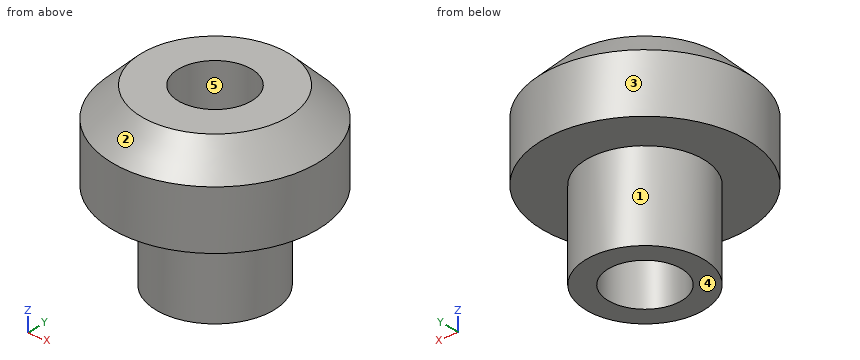
Solid Edge part; units mm, degrees
sketch "Sketch1" plane through (0, 0, 0) normal (0, 0, 1) x (1, 0, 0)
  circle A0 centre (0, 0) radius 1.25
  circle A1 centre (0, 0) radius 2
extrude "Protrusion1" add sketch "Sketch1" along normal blind 3
sketch "Sketch2" plane through (0, 0, 3) normal (0, 0, 1) x (1, 0, 0)
  circle A0 centre (0, 0) radius 1.25
  circle A1 centre (0, 0) radius 3.5
extrude "ExtrudedProtrusion_2" add sketch "Sketch2" along normal blind 3
chamfer "Chamfer_1" distance 1 angle 45 1 edges at (-3.5, 0, 6)
properties material "ABS Plastic, medium impact"
Check sheet for the modelled part. Datum: model origin and axes. Units: mm. Face numbers are marked on the shaded views. A direction names the side the tool comes from. Give positions to 0.01 mm unless a question says otherwise; leave off trailing zeros. Write each loop counter-clockwise with the first axis right and the second up, starting at its lowest first coordinate (ties: lowest second). Pieces come first, ordered by that corner, then holes. Notation, with made-up numbers: M 0.5,29.25 L 22.5,29.25 A21 cw 22.5,37.25 Z; hole C 30,-18.5 d7. An arc over 180 degrees is marked long. Use one line per item in the form item = value.
(1) Depth check by flat-ended pin: P1, Ø2, axis at x = 1, y = -1, coming from the -Z side; P2, Ø2, axis at y = 2, z = 1.5, coming from the -X side; P3, Ø2, axis at x = 1.5, z = 4, coming from the -Y side. Enter the tip coordinate at first touch or a pass-through.
Answer block:
P1 = 0
P2 = -1.73
P3 = -3.46
(2) Section check C-C on z = 3.35. Record the boundary of the cut face in (x, y), plus the area to 3 significant figures.
Answer block:
outline = C 0,0 d7; hole C 0,0 d2.5
area = 33.6 mm2
(3) Material ranges on line 1 along Y through (x, z) = (0, 4.7); line 2 along Y through (x, z) = (0, 2); line 3 along X through (y, z) = (0.5, 1.75), recorded low to high.
Answer block:
line_1 = -3.5 to -1.25, 1.25 to 3.5
line_2 = -2 to -1.25, 1.25 to 2
line_3 = -1.94 to -1.15, 1.15 to 1.94
(4) Section check D-D on z = 1.75. Record the boundary of the cut face in (x, y), plus the area to 3 significant figures.
Answer block:
outline = C 0,0 d4; hole C 0,0 d2.5
area = 7.66 mm2
(5) Section check A-A on y = 0. Record the boundary of the cut face in (x, z).
Answer block:
outline = M -3.5,3 L -2,3 L -2,0 L -1.25,0 L -1.25,6 L -2.5,6 L -3.5,5 Z; M 1.25,0 L 2,0 L 2,3 L 3.5,3 L 3.5,5 L 2.5,6 L 1.25,6 Z
(6) Tool access check on the marked faces 1 and 2. Record the directions out of +Z, -Z, +X, -X, +Y, -Y that give a thin tool (end or side, any length) a straight path to the whole face; none if there is none.
Answer block:
face_1 = -Z
face_2 = +Z
(7) Draft check along Y on the marked faces 3, 4 and 5. Enter one of: pulls with the +Y half, pulls with the -Y half, needs draft (parallel to the pull), parting line crosses it, or undercut.
Answer block:
face_3 = parting line crosses it
face_4 = needs draft
face_5 = undercut
